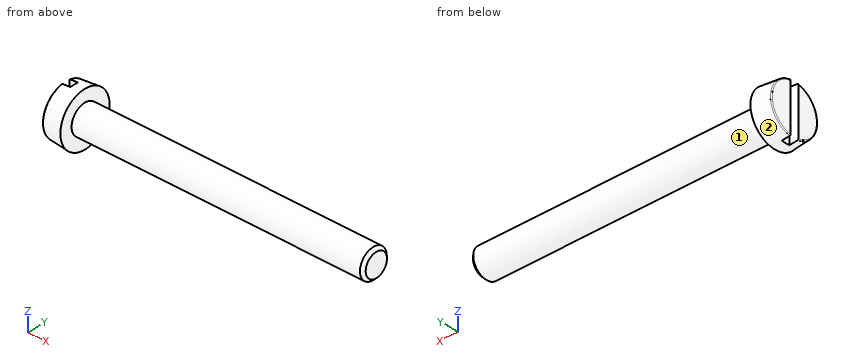
Autodesk Inventor part; units mm, degrees
ref_plane "Work Plane1" through (30.1625, 0, 0) normal (0, 0, -1) x (1, 0, 0)
ref_plane "YZ Plane" through (0, 0, 0) normal (1, 0, 0) x (0, 1, 0)
ref_plane "XZ Plane" through (0, 0, 0) normal (0, 1, 0) x (-1, 0, 0)
sketch "Esquisse1" plane through (0, 0, 0) normal (0, 0, 1) x (1, 0, 0)
  line L0 (-2, 0) -> (30, 0)
  line L1 (30, 0) -> (30, 1.5)
  line L2 (30, 1.5) -> (18, 1.5)
  line L3 (18, 1.5) -> (17.6932, 1.5)
  line L4 (17.6932, 1.5) -> (0, 1.5)
  line L5 (0, 1.5) -> (0, 2.75)
  line L6 (-8.4, 0) -> (36.4, 0)
  line L7 (0, -0.55) -> (0, 3.3)
  line L8 (-2, 0) -> (-2, 2.575)
  line L9 (0, 2.75) -> (-2, 2.575)
  line L10 (18, 1.5) -> (0, 1.5) construction
  dimension "d0" = 30
  dimension "d1" = 12
  dimension "d2" = 0.3068
  dimension "d3" = 2
  dimension "d4" = 3
  dimension "d5" = 3
  dimension "d9" = 5.5
  dimension "d10" = 5
revolve "Corps" add sketch "Esquisse1" angle 360 about axis through (-2, 0, 0) along (1, 0, 0)
sketch "Esquisse2" plane through (-2, 0, 0) normal (-1, 0, 0) x (0, 0, 1)
  circle A0 centre (0, 0) radius 2.75
  line L0 (0, 0) -> (0, 2.575)
  line L1 (-2.75, 0.43) -> (2.75, 0.43)
  line L2 (2.75, 0.43) -> (2.75, -0.43)
  line L3 (2.75, -0.43) -> (-2.75, -0.43)
  line L4 (-2.75, -0.43) -> (-2.75, 0.43)
  line L5 (-2.75, 0) -> (2.75, 0) construction
  line L6 (0, 0.43) -> (0, -0.43) construction
  dimension "d11" = 0.86
  dimension "d12" = 5.5
fillet "Congé1" radius 0.1 1 edges at (-2, -2.575, 0)
extrude "Rainure" cut sketch "Esquisse2" against normal blind 0.9 contours A0 L3 L1 | L2 L3 A0 | A0 L1 L2 | A0 L4 L1 | L3 L4 A0
thread "Filetage"
chamfer "Chanfrein1" distance 0.3067 distance2 0.3068 1 edges at (30, -1.5, 0) measured on face at (30, 0.3888, 0.4512)
ref_plane "Work Plane1" through (30.1625, 0, 0) normal (0, 0, -1) x (1, 0, 0)
equation "\"d11\" = SBR"
equation "\"d12\" = KOD"
equation "\"d14\" = RR"
equation "\"d19\" = STI"
equation "\"d15\" = GEL"
equation "\"d17\" = -0.5 * SPD + 0.5 * GD"
equation "\"d0\" = NLG"
equation "\"d1\" = GEL"
equation "\"d3\" = KOH"
equation "\"d4\" = GD"
equation "\"d5\" = BDM"
equation "\"d9\" = KOD"
equation "\"d10\" = KEWI"
equation "\"GD\" = NND"
equation "\"NLG\" = 30"
equation "\"GEL\" = 12"
equation "\"KOD\" = 5.5"
equation "\"KOH\" = 2"
equation "\"GAL\" = 0.61345 * PTC"
equation "\"SPD\" = NND - 1.2269 * PTC"
equation "\"BDM\" = NND"
equation "\"GUL\" = 0.61345 * PTC"
equation "\"RR\" = 0.1"
equation "\"SBR\" = 0.86"
equation "\"STI\" = 0.9"
equation "\"KEWI\" = 5deg"
equation "\"PTC\" = 0.5"
equation "\"THREADDIA\" = 3"
equation "\"TOA\" = 30deg"
equation "\"NND\" = 3"
equation "\"GD1\" = THREADDIA - 1.2269 * PTC"
properties part number "CSN 02 1131 - M3 x 30" material "Acier, doux"
Design review of the part built by this model. Coordinates are the model's own, in mm. Face numbers are marked on the shaded views. A direction names the side the tool comes from. Coordinates: 2 decimals unless noted, no trailing zeros. Loops run counter-clockwise (first coordinate to the right, second up) from the corner with the lowest first, then second, coordinate; pieces in that order, holes last. Notation, with made-up numbers: (-27.5, 57.25) - (-7.5, 57.25) arc R29 ccw to (-7.5, 85.25) - close; hole circle Ø11 at (82.25, 23.5). An arc over 180 degrees is marked (long way). Use CSV: the item, a comma, the result in double quotes. Start each with the question number.
1. To check wall thickness, follow probe 1 along X at (y, z) = (-1.7, -1.3); probe 2 along Z at (x, y) = (4, -0.05); probe 3 along Y at (x, z) = (14, -0.9). State the ranges of each line that lie inside material, in increasing order.
2. Clearance check with flat-ended pins moving along their axes: pin 1 (2 mm diameter, centred on x = 15.5, y = 1.5, fed in from +Z); pin 2 (0.7 mm diameter, centred on y = 0, z = -0.5, fed in from -X); pin 3 (0.5 mm diameter, centred on x = -1.5, z = 0.5, fed in from -Y). State where each tip first meets the part, or that it passes through.
3. Add section C-C on x = 5.5. Give the boundary of the cut face in (y, z), plus the area to 3 significant figures.
4. For the marked faces 1 and 2, list the 3-axis set-ups (+Z, -Z, +X, -X, +Y, -Y) from which the entire face can be reached by the end or side of a thin tool; tool diameter is ignored.
5. Add section B-B on z = 0. Give the boundary of the cut face in (x, y), plus the area to 3 significant figures.
6. Add section A-A on y = 0. Give the boundary of the cut face in (x, z).
Resolved:
1,probe 1,"-2 to 0"
1,probe 2,"-1.5 to 1.5"
1,probe 3,"-1.2 to 1.2"
2,pin 1,"z = 1.41"
2,pin 2,"x = -1.1"
2,pin 3,"y = -2.61"
3,outline,"circle Ø3 at (0, 0)"
3,area,"7.07 mm2"
4,face 1,"+X"
4,face 2,"-X"
5,outline,"(-2, -2.48) arc R0.1 ccw to (-1.91, -2.58) - (0, -2.75) - (0, -1.5) - (29.69, -1.5) - (30, -1.19) - (30, 1.19) - (29.69, 1.5) - (0, 1.5) - (0, 2.75) - (-1.91, 2.58) arc R0.1 ccw to (-2, 2.48) - (-2, 0.43) - (-1.1, 0.43) - (-1.1, -0.43) - (-2, -0.43) - close"
5,area,"99.8 mm2"
6,outline,"(-1.1, -2.65) - (0, -2.75) - (0, -1.5) - (29.69, -1.5) - (30, -1.19) - (30, 1.19) - (29.69, 1.5) - (0, 1.5) - (0, 2.75) - (-1.1, 2.65) - close"
